Autodesk Inventor part; units mm, degrees
ref_plane "YZ Plane" through (0, 0, 0) normal (1, 0, 0) x (0, 1, 0)
ref_plane "XZ Plane" through (0, 0, 0) normal (0, 1, 0) x (-1, 0, 0)
ref_plane "XY Plane" through (0, 0, 0) normal (0, 0, 1) x (1, 0, 0)
sketch "Szkic1" plane through (0, 0, 0) normal (0, 1, 0) x (-1, 0, 0)
  line L0 (-101.5, -209) -> (101.5, -209)
  line L1 (101.5, -209) -> (101.5, 209)
  line L2 (101.5, 209) -> (-101.5, 209)
  line L3 (-101.5, 209) -> (-101.5, -209)
  line L4 (-101.5, -209) -> (101.5, 209) construction
  line L5 (101.5, -209) -> (-101.5, 209) construction
  line L6 (-101.5, -94) -> (58.5, -94)
  line L7 (58.5, -94) -> (58.5, -14)
  line L8 (58.5, -14) -> (-101.5, -14)
  line L9 (-101.5, -14) -> (-101.5, -94)
  circle A0 centre (76.5, 157) radius 6.1
  point P0 (0, 0)
  dimension "d0" = 203
  dimension "d1" = 418
  dimension "d2" = 160
  dimension "d3" = 80
  dimension "d4" = 115
  dimension "d5" = 12.2
  dimension "d6" = 25
  dimension "d7" = 52
extrude "Wyciągnięcie proste1" add sketch "Szkic1" along normal mid plane 3 contours L3 L6 L7 L8 L2 L1 L0
properties part number "scina_fronotwa"
Geometry check sheet. Reference: the model listing, model coordinates, mm. Give positions to 0.01 mm unless a question says otherwise; leave off trailing zeros. Order: outer loops, then holes, each group sorted by start corner. A loop starts at its lowest first (then second) coordinate and runs counter-clockwise, first axis right, second up.
1) Draft check along Z on faces 1 (the cylindrical face through (-82.135, -0.021, 159.336)), 2 (the flat face through (1, -1.5, 3)). Enter one of: released by +Z, released by -Z, zero draft, split by the parting line, or undercut.
Results are:
face 1: undercut
face 2: zero draft
2) Material ranges on probe 1 along Z at (x, y) = (-76.5, -0.75); probe 2 along Z at (x, y) = (-10, -1.3), recorded low to high.
Results are:
probe 1: z = -209 to 150.9, 163.1 to 209
probe 2: z = -209 to -94, -14 to 209
3) Gauge pin test, flat end, axial feed: pin 1 (19.5 mm diameter, centred on x = -76.5, z = 157, fed in from +Y). Record the tip position at first contact, or that the pin passes through.
Results are:
pin 1: stops at y = 1.5
4) Cross-section at C-C (y = 0.85). Record the boundary of the cut face in (x, z), then the cut area to 3 significant figures.
Results are:
outline: (-101.5, -209) - (101.5, -209) - (101.5, -94) - (-58.5, -94) - (-58.5, -14) - (101.5, -14) - (101.5, 209) - (-101.5, 209) - close; hole circle Ø12.2 at (-76.5, 157)
area: 71,900 mm2
5) Cross-section at A-A (x = 9.5). Record the boundary of the cut face in (y, z), then the cut area to 3 significant figures.
Results are:
outline: (-1.5, -209) - (1.5, -209) - (1.5, -94) - (-1.5, -94) - close; (-1.5, -14) - (1.5, -14) - (1.5, 209) - (-1.5, 209) - close
area: 1,010 mm2
6) Cross-section at B-B (z = 157). Record the boundary of the cut face in (x, y), then the cut area to 3 significant figures.
Results are:
outline: (-101.5, -1.5) - (-82.6, -1.5) - (-82.6, 1.5) - (-101.5, 1.5) - close; (-70.4, -1.5) - (101.5, -1.5) - (101.5, 1.5) - (-70.4, 1.5) - close
area: 572 mm2
7) Cross-section at D-D (z = -84). Record the boundary of the cut face in (x, y), then the cut area to 3 significant figures.
Results are:
outline: (-101.5, -1.5) - (-58.5, -1.5) - (-58.5, 1.5) - (-101.5, 1.5) - close
area: 129 mm2
